from build123d import *

# Parameters (mm, degrees)
F0_R     = 80
F0_R_2   = 5
F0_R_3   = 2.25
F1_DEPTH = 2.5
F2_R     = 5


with BuildPart() as f1:
    # F0 (on Right) → F1 (new body)
    with BuildSketch(Plane.YZ):
        Circle(F0_R)
        with BuildLine():
            ThreePointArc((-64.226163, 10), (0, 65), (64.226163, 10))
            ThreePointArc((64.226163, 10), (64.806252, 5.014948), (65, 0))
            ThreePointArc((65, 0), (64.806252, -5.014948), (64.226163, -10))
            ThreePointArc((64.226163, -10), (0, -65), (-64.226163, -10))
            ThreePointArc((-64.226163, -10), (-65, 0), (-64.226163, 10))
        make_face(mode=Mode.SUBTRACT)
        with BuildLine():
            ThreePointArc((-11.18034, -10), (-15, 0), (-11.18034, 10))
            Line((-11.18034, 10), (-64.226163, 10))
            ThreePointArc((-64.226163, 10), (-65, 0), (-64.226163, -10))
            Line((-64.226163, -10), (-11.18034, -10))
        make_face()
        with Locations((-25.75, 0)):
            Circle(F0_R_2, mode=Mode.SUBTRACT)
        with BuildLine():
            ThreePointArc((11.18034, -10), (14.012585, -5.352331), (15, 0))
            ThreePointArc((15, 0), (14.012585, 5.352331), (11.18034, 10))
            ThreePointArc((11.18034, 10), (0, 15), (-11.18034, 10))
            ThreePointArc((-11.18034, 10), (-15, 0), (-11.18034, -10))
            ThreePointArc((-11.18034, -10), (0, -15), (11.18034, -10))
        make_face()
        Circle(F0_R_3, mode=Mode.SUBTRACT)
        with BuildLine():
            ThreePointArc((11.18034, 10), (14.012585, 5.352331), (15, 0))
            ThreePointArc((15, 0), (14.012585, -5.352331), (11.18034, -10))
            Line((11.18034, -10), (64.226163, -10))
            ThreePointArc((64.226163, -10), (64.806252, -5.014948), (65, 0))
            ThreePointArc((65, 0), (64.806252, 5.014948), (64.226163, 10))
            Line((64.226163, 10), (11.18034, 10))
        make_face()
        with Locations((25.75, 0)):
            Circle(F0_R_2, mode=Mode.SUBTRACT)
    extrude(amount=F1_DEPTH)

    # F2
    f2_edges = [f1.edges().sort_by_distance(p)[0] for p in [
        (1.25, -64.226163, 10),
        (1.25, -11.18034, 10),
        (1.25, 11.18034, 10),
        (1.25, 64.226163, 10),
        (1.25, 64.226163, -10),
        (1.25, 11.18034, -10),
        (1.25, -11.18034, -10),
        (1.25, -64.226163, -10),
    ]]
    fillet(f2_edges, radius=F2_R)


solid = f1.part
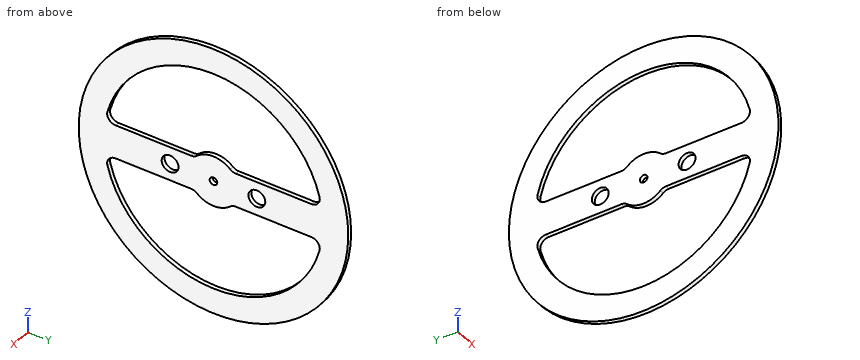
Read the model definition and answer for the solid it produces. Units are mm, in the model's axes. Round coordinates to 2 decimals unless told otherwise and drop trailing zeros. Write each loop counter-clockwise with the first axis right and the second up, starting at its lowest first coordinate (ties: lowest second). Pieces come first, ordered by that corner, then holes.
1. The part is cut by section B-B, the plane y = 0. Determine the outline of the cut face in (x, z), then the cut area to 3 significant figures.
2. The part is cut by section C-C, the plane x = 0.45. Determine the outline of the cut face in (y, z).
3. The part is cut by section D-D, the plane z = -44.5. Determine the outline of the cut face in (x, y).
4. The part is cut by section A-A, the plane z = 0. Determine the outline of the cut face in (x, y), then the cut area to 3 significant figures.
5. Given pin 1 Ø1.2 at (x, y) = (1, 37) entering from -Z; pin 2 Ø0.8 at (x, y) = (2, -33.5) entering from -Z; pin 3 Ø1.2 at (x, y) = (1.5, 37) entering from +Z, each flat-ended and moving along its own axis, determine where each tip first touches the part or whether it passes through.
6. Straight lines are drawn through the part: L1, parallel to Z at x = 1.2, y = 25.75; L2, parallel to Z at x = 1.1, y = -49; L3, parallel to Z at x = 0.95, y = -43. For each, find the intervals that lie inside material, in ascending order.
Values:
1. outline: (0, -80) - (2.5, -80) - (2.5, -65) - (0, -65) - close; (0, -15) - (2.5, -15) - (2.5, -2.25) - (0, -2.25) - close; (0, 2.25) - (2.5, 2.25) - (2.5, 15) - (0, 15) - close; (0, 65) - (2.5, 65) - (2.5, 80) - (0, 80) - close
1. area: 139 mm2
2. outline: circle Ø160 at (0, 0); hole (-62.94, -16.25) arc R65 ccw to (62.94, -16.25) arc R5 ccw to (58.09, -10) - (13.23, -10) arc R5 ccw to (9.92, -11.25) arc R15 cw to (-9.92, -11.25) arc R5 ccw to (-13.23, -10) - (-58.09, -10) arc R5 ccw to start; hole (-62.94, 16.25) arc R5 ccw to (-58.09, 10) - (-13.23, 10) arc R5 ccw to (-9.92, 11.25) arc R15 cw to (9.92, 11.25) arc R5 ccw to (13.23, 10) - (58.09, 10) arc R5 ccw to (62.94, 16.25) arc R65 ccw to start; hole circle Ø10 at (-25.75, 0); hole circle Ø4.5 at (0, 0); hole circle Ø10 at (25.75, 0)
3. outline: (0, -66.48) - (2.5, -66.48) - (2.5, -47.38) - (0, -47.38) - close; (0, 47.38) - (2.5, 47.38) - (2.5, 66.48) - (0, 66.48) - close
4. outline: (0, -80) - (2.5, -80) - (2.5, -30.75) - (0, -30.75) - close; (0, -20.75) - (2.5, -20.75) - (2.5, -2.25) - (0, -2.25) - close; (0, 2.25) - (2.5, 2.25) - (2.5, 20.75) - (0, 20.75) - close; (0, 30.75) - (2.5, 30.75) - (2.5, 80) - (0, 80) - close
4. area: 339 mm2
5. pin 1: stops at z = -71.24
5. pin 2: stops at z = -72.83
5. pin 3: stops at z = 71.24
6. L1: z = -75.74 to -59.68, -10 to -5, 5 to 10, 59.68 to 75.74
6. L2: z = -63.24 to -42.71, -10 to 10, 42.71 to 63.24
6. L3: z = -67.46 to -48.74, -10 to 10, 48.74 to 67.46
